Design review of the part shown in the three views and the two pictorial views. Dimensions are in mm from the part's minimum x, y and z. Round coordinates to 2 decimals unless told otherwise and drop trailing zeros. Order: outer loops, then holes, each group sorted by start corner. A loop starts at its lowest first (then second) coordinate and runs counter-clockwise, first axis right, second up. Notation, with made-up numbers: M 8.25,-25 L 28.25,-25 A33 cw 28.25,5 Z; hole C 33.25,-3.5 d11. An arc over 180 degrees is marked long. Use a Markdown table: item, result. Add a question column.
(1) Take a section at C-C (y = 0.65). Write out the cut boundary in (x, z) (1 decimal), then the cut area to 3 significant figures.
(2) Take a section at B-B (x = 15.24). Write out the cut boundary in (y, z) (1 decimal).
(3) To check wall thickness, follow probe 1 along X at (y, z) = (0.95, 3.81); probe 2 along Z at (x, y) = (25.5, 0.45) (1 decimal); probe 3 along X at (y, z) = (0.35, 4). State the ranges of each line that lie inside material, in increasing order. Write a range as from..to.
(4) For pin 1 (3 mm diameter, centred on x = 25.4, z = 3.81, fed in from +Y); pin 2 (4 mm diameter, centred on x = 25.4, z = 34.29, fed in from +Y), all flat-tipped, find the tip position at first contact; note any pin that passes through.
(5) Take a section at D-D (x = 25.4). Write out the cut boundary in (y, z).
(6) The part is to be moulded in two halves that separate along Y. For the marked faces 1 and 2, say which applies: released by +Y, released by -Y, zero draft, split by the parting line, or undercut.
(7) Take a section at A-A (z = 34.29). Write out the cut boundary in (x, y).
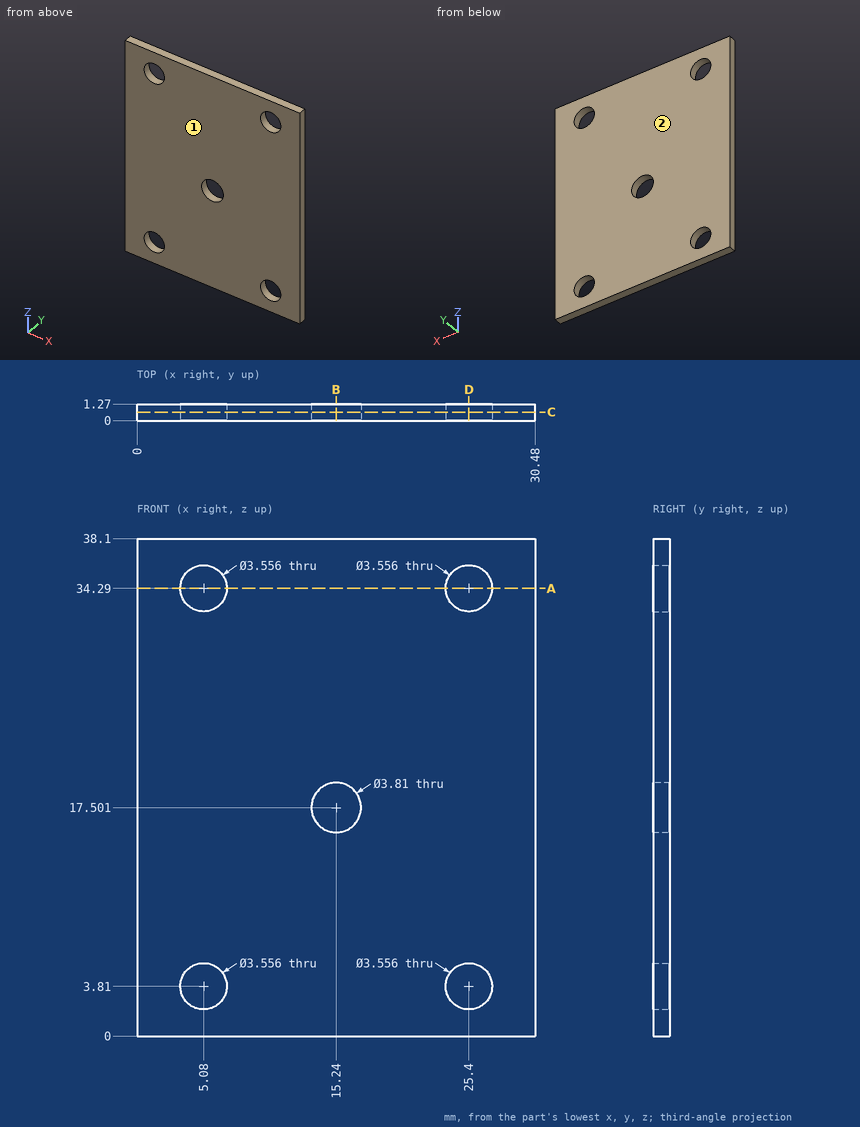
Verdict:
| question | item | result |
|---|---|---|
| 1 | outline | M 0,0 L 30.5,0 L 30.5,38.1 L 0,38.1 Z; hole C 5.1,3.8 d3.6; hole C 5.1,34.3 d3.6; hole C 15.2,17.5 d3.8; hole C 25.4,3.8 d3.6; hole C 25.4,34.3 d3.6 |
| 1 | area | 1,110 mm^2 |
| 2 | outline | M 0,0 L 1.3,0 L 1.3,15.6 L 0,15.6 Z; M 0,19.4 L 1.3,19.4 L 1.3,38.1 L 0,38.1 Z |
| 3 | probe 1 | x = 0..3.3, 6.86..23.62, 27.18..30.48 |
| 3 | probe 2 | z = 0..2, 5.6..32.5, 36.1..38.1 |
| 3 | probe 3 | x = 0..3.31, 6.85..23.63, 27.17..30.48 |
| 4 | pin 1 | passes through |
| 4 | pin 2 | stops at y = 1.27 |
| 5 | outline | M 0,0 L 1.27,0 L 1.27,2.03 L 0,2.03 Z; M 0,5.59 L 1.27,5.59 L 1.27,32.51 L 0,32.51 Z; M 0,36.07 L 1.27,36.07 L 1.27,38.1 L 0,38.1 Z |
| 6 | face 1 | released by -Y |
| 6 | face 2 | released by +Y |
| 7 | outline | M 0,0 L 3.3,0 L 3.3,1.27 L 0,1.27 Z; M 6.86,0 L 23.62,0 L 23.62,1.27 L 6.86,1.27 Z; M 27.18,0 L 30.48,0 L 30.48,1.27 L 27.18,1.27 Z |
